Here's how the part is built. I have some questions about the finished solid (model axes, mm). A direction names the side the tool comes from. Round coordinates to 2 decimals unless told otherwise and drop trailing zeros. Order: outer loops, then holes, each group sorted by start corner. A loop starts at its lowest first (then second) coordinate and runs counter-clockwise, first axis right, second up. Notation, with made-up numbers: (80.5, -15.75) - (92.5, -15.75) arc R29 cw to (92.5, 22.25) - close; hole circle Ø5 at (47, 76). An arc over 180 degrees is marked (long way). Answer as a JSON object with one key per item and string values.
```python
from build123d import *

# Parameters (mm, degrees)
SKETCH1_R             = 19.5
SKETCH1_R_2           = 8.15
SKETCH1_R_3           = 6.65
SKETCH1_R_4           = 5.15
DISCO_SEPARADOR_DEPTH = 4
SKETCH2_W             = 7
SKETCH2_H             = 10
PATA_AL_HUESO_DEPTH   = 4


with BuildPart() as part:
    # Sketch1 → Disco_separador (new body)
    with BuildSketch(Plane(origin=(0, -2, 0), x_dir=(1, 0, 0), z_dir=(0, 1, 0))):
        with Locations(Location((0, 0, 0), (0, 0, 270))):
            Circle(SKETCH1_R)
        with Locations(Location((-8.5, 0, 0), (0, 0, 270))):
            Circle(SKETCH1_R_2, mode=Mode.SUBTRACT)
        with Locations(Location((4, -9.5, 0), (0, 0, 270))):
            Circle(SKETCH1_R_3, mode=Mode.SUBTRACT)
        with Locations(Location((4, 9.5, 0), (0, 0, 270))):
            Circle(SKETCH1_R_3, mode=Mode.SUBTRACT)
        with Locations(Location((13.5, 0, 0), (0, 0, 270))):
            Circle(SKETCH1_R_4, mode=Mode.SUBTRACT)
    extrude(amount=DISCO_SEPARADOR_DEPTH)

    # Sketch2 → Pata_al_hueso (add)
    with BuildSketch(Plane(origin=(0, -2, 0), x_dir=(1, 0, 0), z_dir=(0, 1, 0))):
        with Locations((-21, 0)):
            Rectangle(SKETCH2_W, SKETCH2_H)
    extrude(amount=PATA_AL_HUESO_DEPTH)


solid = part.part
```
1. Imagine slicing it at C-C (y = 0.65). List the corners of the cut face in (x, z) for me, plus the area to 3 significant figures.
Responses:
{"outline": "(-24.5, -5) - (-18.85, -5) arc R19.5 ccw (long way) to (-18.85, 5) - (-24.5, 5) - close; hole circle Ø16.3 at (-8.5, 0); hole circle Ø13.3 at (4, -9.5); hole circle Ø13.3 at (4, 9.5); hole circle Ø10.3 at (13.5, 0)", "area": "677 mm2"}
2. Imagine slicing it at A-A (z = 0). List the corners of the cut face in (x, y) for me, plus the area to 3 significant figures.
Responses:
{"outline": "(-24.5, -2) - (-16.65, -2) - (-16.65, 2) - (-24.5, 2) - close; (-0.35, -2) - (8.35, -2) - (8.35, 2) - (-0.35, 2) - close; (18.65, -2) - (19.5, -2) - (19.5, 2) - (18.65, 2) - close", "area": "69.6 mm2"}
3. If I drill on L1, parallel to X at y = -0.5, z = 0; L2, parallel to X at y = 1.7, z = -4.5; L3, parallel to X at y = -1.1, z = 4, over which ranges is the centre line in solid material (lowest first)? Write a range as [from, to].
Responses:
{"L1": "[-24.5, -16.65], [-0.35, 8.35], [18.65, 19.5]", "L2": "[-24.5, -15.3], [-1.7, -0.38], [8.38, 11], [16, 18.97]", "L3": "[-24.5, -15.6], [-1.4, 0.26], [7.74, 10.26], [16.74, 19.09]"}
4. Imagine slicing it at D-D (z = -13). List the corners of the cut face in (x, y) for me, plus the area to 3 significant figures.
Responses:
{"outline": "(-14.53, -2) - (-1.65, -2) - (-1.65, 2) - (-14.53, 2) - close; (9.65, -2) - (14.53, -2) - (14.53, 2) - (9.65, 2) - close", "area": "71.0 mm2"}
5. Imagine slicing it at B-B (x = -5). List the corners of the cut face in (y, z) for me, plus the area to 3 significant figures.
Responses:
{"outline": "(-2, -18.85) - (2, -18.85) - (2, -7.36) - (-2, -7.36) - close; (-2, 7.36) - (2, 7.36) - (2, 18.85) - (-2, 18.85) - close", "area": "91.9 mm2"}
6. Thinking about a two-plate mould opening in X: for faces 1 (the face through (-24.5, 0, 0)), 2 (the face through (19.484, -0.028, 0.787)), 3 (the face through (2, 2, 0)), 4 (the face through (-16.456, -0.028, -1.767)), which applies, pulls with the +X half, pulls with the -X half, needs draft (parallel to the pull), parting line crosses it, or undercut?
Responses:
{"face 1": "pulls with the -X half", "face 2": "parting line crosses it", "face 3": "needs draft", "face 4": "undercut"}
7. For faces 5 (the face through (-22, 0, -5)), 6 (the face through (-22, 0, 5)), 7 (the face through (5.997, -0.028, -3.157)), which set-ups out of +Z, -Z, +X, -X, +Y, -Y let a thin tool reach every point of the face, with its end or its side?
Responses:
{"face 5": "-Z, -X, +Y, -Y", "face 6": "+Z, -X, +Y, -Y", "face 7": "+Y, -Y"}
8. For P1, Ø1.5, axis at y = 1, z = 12.5, coming from the +X side, with a flat end and sliding along its axis, tell me the tip position at first contact or that it passes through.
Responses:
{"P1": "x = 15.56"}
